Solid Edge part; units mm, degrees
sketch "Sketch1" plane through (0, 0, 0) normal (0, -1, 0) x (1, 0, 0)
  line L0 (0, 0) -> (60, 0)
  line L1 (60, 0) -> (60, -95)
  line L2 (60, -95) -> (40, -95)
  line L3 (40, -95) -> (40, -15)
  line L4 (40, -15) -> (-40, -15)
  line L5 (-40, -15) -> (-40, -95)
  line L6 (-40, -95) -> (-60, -95)
  line L7 (-60, -95) -> (-60, 0)
  line L8 (-60, 0) -> (0, 0)
extrude "Protrusion1" add sketch "Sketch1" along normal mid plane 80
sketch "Sketch2" plane through (60, 0, -47.5) normal (1, 0, 0) x (0, 1, 0)
  circle A0 centre (0, -7.5) radius 15
extrude "ExtrudedCutout_1" cut sketch "Sketch2" against normal blind 120
fillet "Round_3" radius 40 4 edges at (50, -40, -95) (50, 40, -95) (-50, 40, -95) (-50, -40, -95)
sketch "Sketch3" plane through (0, 0, 0) normal (0, 0, 1) x (1, 0, 0)
  circle A0 centre (0, 0) radius 40
extrude "ExtrudedProtrusion_3" add sketch "Sketch3" along normal blind 20
sketch "Sketch4" plane through (0, 0, 20) normal (0, 0, 1) x (1, 0, 0)
  circle A0 centre (0, 0) radius 30
extrude "ExtrudedCutout_3" cut sketch "Sketch4" against normal blind 15
sketch "Sketch5" plane through (0, 0, 5) normal (0, 0, 1) x (1, 0, 0)
  circle A0 centre (0, 0) radius 15
extrude "ExtrudedCutout_4" cut sketch "Sketch5" against normal blind 20
The listing builds one solid part. Answer for the finished solid, in the listing's coordinates (mm). A direction names the side the tool comes from. Round coordinates to 2 decimals unless told otherwise and drop trailing zeros. Write each loop counter-clockwise with the first axis right and the second up, starting at its lowest first coordinate (ties: lowest second). Pieces come first, ordered by that corner, then holes. Notation, with made-up numbers: (3, 3.5) -> (27, 3.5) arc R6 ccw to (27, 14.5) -> close; hole circle Ø4 at (18, -14.75). An arc over 180 degrees is marked (long way). Use CSV: the item, a comma, the result in double quotes. Start each with the question number.
(1) The mould has two halves that part along Z. Classify faces 4 (the face through (43, 1, 0)), 5 (the face through (50.14, -3.252, -69.643)), 6 (the face through (49.86, 28.595, -82.973)), 7 (the face through (-49.86, -3.252, -69.643)): released by +Z, released by -Z, zero draft, split by the parting line, or undercut.
(2) Each of these flat-tipped pins is pushed along its axis until it touches: pin 1 (5 mm diameter, centred on x = 43, y = 28, fed in from +Z); pin 2 (12 mm diameter, centred on x = 14.5, y = 23, fed in from -Z). Where does it stop, or does it pass through?
(3) Section B-B on z = -32 is taken. Give the vertices of the cut face in (x, y).
(4) Section D-D on x = 32 is taken. Give the vertices of the cut face in (y, z), then the cut area to 3 significant figures.
(5) Section C-C on z = -59 is taken. Give the vertices of the cut face in (x, y).
(6) Consider L1, parallel to X at y = -33, z = -76; L2, parallel to Y at x = 0, z = 11.25; L3, parallel to Y at x = 0, z = 0. Determine where each line is inside the solid, lowest interval first. Write a range as from..to.
(7) Which of the six approach directions +Z, -Z, +X, -X, +Y, -Y give full straight-line access (tool end or side, diameter ignored) to faces 1 (the face through (40, 1, -38)), 2 (the face through (-44, 1, 0)), 3 (the face through (-29.97, 1.32, 12.6))?
A:
1,face 4,"released by +Z"
1,face 5,"undercut"
1,face 6,"released by -Z"
1,face 7,"undercut"
2,pin 1,"stops at z = 0"
2,pin 2,"stops at z = -15"
3,outline,"(-60, -40) -> (-40, -40) -> (-40, 40) -> (-60, 40) -> close; (40, -40) -> (60, -40) -> (60, 40) -> (40, 40) -> close"
4,outline,"(-40, -15) -> (40, -15) -> (40, 0) -> (24, 0) -> (24, 20) -> (-24, 20) -> (-24, 0) -> (-40, 0) -> close"
4,area,"2,160 mm²"
5,outline,"(-60, -39.8) -> (-40, -39.8) -> (-40, -14.46) -> (-60, -14.46) -> close; (-60, 14.46) -> (-40, 14.46) -> (-40, 39.8) -> (-60, 39.8) -> close; (40, -39.8) -> (60, -39.8) -> (60, -14.46) -> (40, -14.46) -> close; (40, 14.46) -> (60, 14.46) -> (60, 39.8) -> (40, 39.8) -> close"
6,L1,"x = -60..-40, 40..60"
6,L2,"y = -40..-30, 30..40"
6,L3,"y = -40..-15, 15..40"
7,face 1,"-Z, +Y, -Y"
7,face 2,"+Z, -X"
7,face 3,"+Z"
